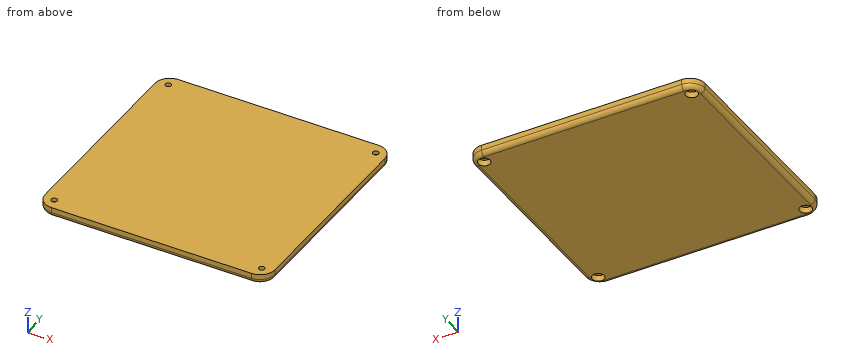
```python
from build123d import *

# Parameters (mm, degrees)
SKETCH1_R           = 1.25
BOSS_EXTRUDE1_DEPTH = 6.5
SKETCH2_R           = 2
CUT_EXTRUDE1_DEPTH  = 334.604931019
FILLET1_R           = 3
SKETCH3_R           = 4
CUT_EXTRUDE2_DEPTH  = 4


with BuildPart() as part:
    # Sketch1 → Boss-Extrude1 (new body)
    with BuildSketch(Plane.XY):
        with BuildLine():
            Line((-315, -75), (-180, -75))
            ThreePointArc((-180, -75), (-172.928932188, -72.071067812), (-170, -65))
            Line((-170, -65), (-170, 65))
            ThreePointArc((-170, 65), (-172.928932188, 72.071067812), (-180, 75))
            Line((-180, 75), (-315, 75))
            ThreePointArc((-315, 75), (-322.071067812, 72.071067812), (-325, 65))
            Line((-325, 65), (-325, -65))
            ThreePointArc((-325, -65), (-322.071067812, -72.071067812), (-315, -75))
        make_face()
        with Locations(Location((-317.5, -67.5, 0), (0, 0, 180))):
            Circle(SKETCH1_R, mode=Mode.SUBTRACT)
        with Locations(Location((-177.5, -67.5, 0), (0, 0, 180))):
            Circle(SKETCH1_R, mode=Mode.SUBTRACT)
        with Locations(Location((-177.5, 67.5, 0), (0, 0, 180))):
            Circle(SKETCH1_R, mode=Mode.SUBTRACT)
        with Locations(Location((-317.5, 67.5, 0), (0, 0, 180))):
            Circle(SKETCH1_R, mode=Mode.SUBTRACT)
    extrude(amount=BOSS_EXTRUDE1_DEPTH)

    # Sketch2 → Cut-Extrude1 (cut, through all)
    with BuildSketch(Plane(origin=(0, 0, 0), x_dir=(-1, 0, 0), z_dir=(0, 0, -1))):
        with Locations((177.5, 67.5)):
            Circle(SKETCH2_R)
        with Locations((317.5, 67.5)):
            Circle(SKETCH2_R)
        with Locations((317.5, -67.5)):
            Circle(SKETCH2_R)
        with Locations((177.5, -67.5)):
            Circle(SKETCH2_R)
    extrude(amount=-CUT_EXTRUDE1_DEPTH, mode=Mode.SUBTRACT)

    # Fillet1
    fillet1_edges = [part.edges().sort_by_distance(p)[0] for p in [
        (-170, 0, 0),
        (-172.928932188, -72.071067812, 0),
        (-247.5, -75, 0),
        (-322.071067812, -72.071067812, 0),
        (-325, 0, 0),
        (-322.071067812, 72.071067812, 0),
        (-247.5, 75, 0),
        (-172.928932188, 72.071067812, 0),
    ]]
    fillet(fillet1_edges, radius=FILLET1_R)

    # Sketch3 → Cut-Extrude2 (cut)
    with BuildSketch(Plane(origin=(0, 0, 0), x_dir=(-1, 0, 0), z_dir=(0, 0, -1))):
        with Locations((177.5, 67.5)):
            Circle(SKETCH3_R)
        with Locations((317.5, 67.5)):
            Circle(SKETCH3_R)
        with Locations((177.5, -67.5)):
            Circle(SKETCH3_R)
        with Locations((317.5, -67.5)):
            Circle(SKETCH3_R)
    extrude(amount=-CUT_EXTRUDE2_DEPTH, mode=Mode.SUBTRACT)


solid = part.part
```
Could you check a few things on this model? Use its own coordinates, in mm. Coordinates: 2 decimals unless noted, no trailing zeros. Write each loop counter-clockwise with the first axis right and the second up, starting at its lowest first coordinate (ties: lowest second). Pieces come first, ordered by that corner, then holes. Notation, with made-up numbers: (19, 76.5) -> (28, 76.5) arc R22 ccw to (28, 104.5) -> close; hole circle Ø7 at (-37, 41). An arc over 180 degrees is marked (long way). Write item = value, one per line. Start each with the question number.
(1) I need wall thicknesses on line 1 (Y direction, x = -317.5, z = 2.1); line 2 (X direction, y = -68.5, z = 1.5); line 3 (Y direction, x = -317.5, z = 1.15). Which ranges of each line are inside material? Lowest first, please. Write a range as [from, to].
(2) Will these pins go through, and if not, where does the flat tip stop? pin 1 (2.5 mm diameter, centred on x = -318, y = 66.5, fed in from -Z); pin 2 (4.5 mm diameter, centred on x = -317.5, y = 67.5, fed in from +Z); pin 3 (1 mm diameter, centred on x = -213.5, z = 2, fed in from +Y).
(3) I want a section at A-A (z = 1.75). Please give me the cut outline in (x, y), plus the area to 3 significant figures.
Result set:
q1.line_1 = [-74.54, -71.5], [-63.5, 63.5], [71.5, 74.54]
q1.line_2 = [-323.94, -321.37], [-313.63, -181.37], [-173.63, -171.06]
q1.line_3 = [-74.02, -71.5], [-63.5, 63.5], [71.5, 74.02]
q2.pin_1 = 4
q2.pin_2 = 6.5
q2.pin_3 = 74.96
q3.outline = (-324.73, -65) arc R9.73 ccw to (-315, -74.73) -> (-180, -74.73) arc R9.73 ccw to (-170.27, -65) -> (-170.27, 65) arc R9.73 ccw to (-180, 74.73) -> (-315, 74.73) arc R9.73 ccw to (-324.73, 65) -> close; hole circle Ø8 at (-317.5, -67.5); hole circle Ø8 at (-317.5, 67.5); hole circle Ø8 at (-177.5, -67.5); hole circle Ø8 at (-177.5, 67.5)
q3.area = 22,800 mm2
